from build123d import *

# Parameters (mm, degrees)
F1_DEPTH = 81.8546242
F2_R     = 6.35
F3_DEPTH = 39.37
F4_R     = 35.56
F5_DEPTH = 107.95


# Not quite as in the source:
# - a feature names something its author has since deleted; it is built from what else it names


with BuildPart() as f1:
    # F0 (on Top) → F1 (new body)
    with BuildSketch(Plane.XY):
        with BuildLine():
            Line((33.7800627271, 11.1094987354), (36.4443279242, 11.1094987354))
            ThreePointArc((36.4443279242, 11.1094987354), (0, 38.1), (-36.4443279242, 11.1094987354))
            Line((-36.4443279242, 11.1094987354), (-33.7800627271, 11.1094987354))
            ThreePointArc((-33.7800627271, 11.1094987354), (0, 35.56), (33.7800627271, 11.1094987354))
        make_face()
        with BuildLine():
            ThreePointArc((-36.4443279242, -11.1094987354), (0, -38.1), (36.4443279242, -11.1094987354))
            Line((36.4443279242, -11.1094987354), (33.7800627271, -11.1094987354))
            ThreePointArc((33.7800627271, -11.1094987354), (0, -35.56), (-33.7800627271, -11.1094987354))
            Line((-33.7800627271, -11.1094987354), (-36.4443279242, -11.1094987354))
        make_face()
        with BuildLine():
            Line((36.4443279242, -11.1094987354), (36.4443279242, 11.1094987354))
            Line((36.4443279242, 11.1094987354), (33.7800627271, 11.1094987354))
            ThreePointArc((33.7800627271, 11.1094987354), (35.1121961046, 5.6255919433), (35.56, 0))
            ThreePointArc((35.56, 0), (35.1121961046, -5.6255919433), (33.7800627271, -11.1094987354))
            Line((33.7800627271, -11.1094987354), (36.4443279242, -11.1094987354))
        make_face()
        with BuildLine():
            ThreePointArc((36.4443279242, -11.1094987354), (37.683808817, -5.6160976704), (38.1, 0))
            ThreePointArc((38.1, 0), (37.683808817, 5.6160976704), (36.4443279242, 11.1094987354))
            Line((36.4443279242, 11.1094987354), (36.4443279242, -11.1094987354))
        make_face()
    extrude(amount=F1_DEPTH)

    # F2 (on Right) → F3 (join)
    with BuildSketch(Plane.YZ):
        with Locations((0, 40.9273121)):
            Circle(F2_R)
    extrude(amount=F3_DEPTH)

    # F4 (on Top) → F5 (cut, symmetric)
    with BuildSketch(Plane.XY):
        Circle(F4_R)
    extrude(amount=F5_DEPTH, both=True, mode=Mode.SUBTRACT)


solid = f1.part
Source: CAD feature listing. Evaluate the final solid. Frame: model axes, mm. A direction names the side the tool comes from. Round coordinates to 2 decimals unless told otherwise and drop trailing zeros. Order: outer loops, then holes, each group sorted by start corner. A loop starts at its lowest first (then second) coordinate and runs counter-clockwise, first axis right, second up. Notation, with made-up numbers: (-35, 26) - (5, 26) arc R16 ccw to (5, 39) - close; hole circle Ø10 at (54, 70.25). An arc over 180 degrees is marked (long way). Use a Markdown table: item, result. Add a question column.
1. Section query B-B (x = -16). Return the cut outline in (y, z), then the cut area to 3 significant figures.
2. Section query D-D (y = 1.5). Return the cut outline in (x, z), then the cut area to 3 significant figures.
3. Mould query, pull axis Y, two halves, no side actions, for faces 3 (the flat face through (39.37, 0, 41)), 4 (the flat face through (-35, 11.109, 40)), 5 (the cylindrical face through (38.66, 6.06, 42.83)). Classes: +Y half, -Y half, draft (parallel to the pull), parting line (faces both ways), or undercut.
4. Section query A-A (y = 17). Return the cut outline in (x, z).
5. Line query: probe 1 along X at (y, z) = (-28.5, 15.5); probe 2 along X at (y, z) = (-15.5, 4); probe 3 along Y at (x, z) = (13, 69). Output: solid intervals per line, ascending.
6. Section query C-C (z = 30). Return the cut outline in (x, y), then the cut area to 3 significant figures.
7. First-contact query: pin 1 (8 mm diameter, centred on x = -25.5, y = -17, fed in from +Z); pin 2 (4 mm diameter, centred on x = 30, z = 32, fed in from +Y); pin 3 (4 mm diameter, centred on y = 9.5, z = 15.5, fed in from +X); pin 4 (0.8 mm diameter, centred on x = -34.5, z = 60.5, fed in from +Y). Flat tips, straight axial feed; report the tip coordinate or a pass-through.
8. Set-up query: faces 1 (the flat face through (34, -11, 81.855)), 2 (the flat face through (-35, -11.109, 40)). Return all of +Z, -Z, +X, -X, +Y, -Y with unobstructed straight access to the full face (end or side cutting, diameter ignored); none if empty.
Derived:
| question | item | result |
|---|---|---|
| 1 | outline | (-34.58, 0) - (-31.76, 0) - (-31.76, 81.85) - (-34.58, 81.85) - close; (31.76, 0) - (34.58, 0) - (34.58, 81.85) - (31.76, 81.85) - close |
| 1 | area | 462 mm2 |
| 2 | outline | (35.53, 0) - (38.07, 0) - (38.07, 34.76) - (39.37, 34.76) - (39.37, 47.1) - (38.07, 47.1) - (38.07, 81.85) - (35.53, 81.85) - close |
| 2 | area | 224 mm2 |
| 3 | face 3 | draft |
| 3 | face 4 | undercut |
| 3 | face 5 | parting line |
| 4 | outline | (-34.1, 0) - (-31.23, 0) - (-31.23, 81.85) - (-34.1, 81.85) - close; (31.23, 0) - (34.1, 0) - (34.1, 81.85) - (31.23, 81.85) - close |
| 5 | probe 1 | -25.29 to -21.27, 21.27 to 25.29 |
| 5 | probe 2 | -34.8 to -32, 32 to 34.8 |
| 5 | probe 3 | -35.81 to -33.1, 33.1 to 35.81 |
| 6 | outline | (-36.44, -11.11) arc R38.1 ccw (long way) to (-36.44, 11.11) - (-33.78, 11.11) arc R35.56 cw (long way) to (-33.78, -11.11) - close |
| 6 | area | 530 mm2 |
| 7 | pin 1 | through |
| 7 | pin 2 | y = 25.84 |
| 7 | pin 3 | x = 37.35 |
| 7 | pin 4 | y = 16.99 |
| 8 | face 1 | +Z, +X, -X, +Y, -Y |
| 8 | face 2 | +Z, -Z, -X |
